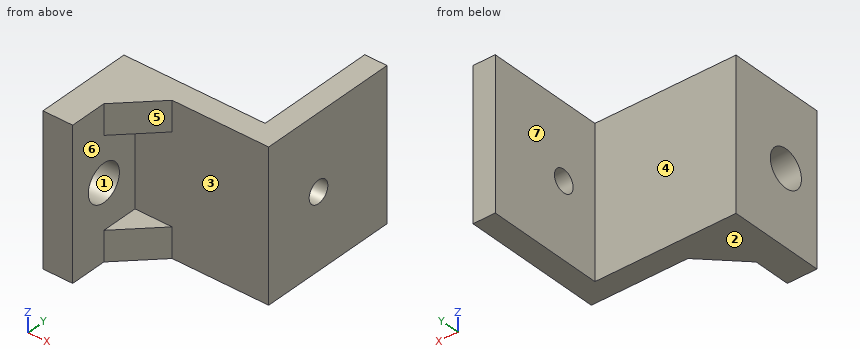
Autodesk Inventor part; units mm, degrees
ref_plane "YZ Plane" through (0, 0, 0) normal (1, 0, 0) x (0, 1, 0)
ref_plane "XZ Plane" through (0, 0, 0) normal (0, 1, 0) x (-1, 0, 0)
ref_plane "XY Plane" through (0, 0, 0) normal (0, 0, 1) x (1, 0, 0)
sketch "Sketch1" plane through (0, 0, 0) normal (0, 0, 1) x (1, 0, 0)
  line L0 (0, 0) -> (22, 0)
  line L1 (22, 0) -> (22, -19)
  line L2 (22, -19) -> (0, -19)
  line L3 (0, -19) -> (0, 0)
  line L4 (3, 0) -> (19, 0)
  line L5 (19, 0) -> (19, -16)
  line L6 (19, -16) -> (3, -16)
  line L7 (3, -16) -> (3, 0)
  dimension "d0" = 22
  dimension "d1" = 19
  dimension "d2" = 3
  dimension "d3" = 3
  dimension "d4" = 3
extrude "Extrusion1" add sketch "Sketch1" along normal blind 20 contours L0 L7 L6 L5 L1 L2 L3
sketch "Sketch4" plane through (3, -16, 0) normal (1, 0, 0) x (0, 0, -1)
  line L0 (-20, 0) -> (-20, 16)
  line L1 (0, 0) -> (-20, 0)
  line L2 (-20, 0) -> (-20, 16)
  line L3 (-20, 16) -> (0, 16)
  line L4 (0, 16) -> (0, 0)
extrude "Extrusion4" cut sketch "Sketch4" against normal through all
sketch "Sketch5" plane through (0, 0, 0) normal (0, 0, -1) x (-1, 0, 0)
  line L0 (0, -19) -> (-22, -19)
  line L1 (0, -19) -> (-4, -19)
  line L2 (-4, -19) -> (-4, -29)
  line L3 (-4, -29) -> (0, -29)
  line L4 (0, -29) -> (0, -19)
  point P0 (0, 0)
  dimension "d17" = 4
  dimension "d18" = 10
extrude "Extrusion5" add sketch "Sketch5" against normal blind 20
sketch "Sketch6" plane through (4, -29, 0) normal (1, 0, 0) x (0, 0, -1)
  line L0 (0, 10) -> (-20, 10)
  line L1 (0, 10) -> (0, 0)
  circle A0 centre (-10, 5) radius 2.5
  point P0 (0, 29)
  dimension "d21" = 5
  dimension "d22" = 10
  dimension "d23" = 5
extrude "Extrusion6" cut sketch "Sketch6" against normal through all
sketch "Sketch7" plane through (0, 0, 0) normal (0, 0, -1) x (-1, 0, 0)
  line L0 (-4, -19) -> (-22, -19)
  line L1 (-4, -29) -> (-4, -19)
  line L2 (-9, -19) -> (-4, -24)
  point P0 (0, 0)
  dimension "d26" = 5
  dimension "d27" = 5
extrude "Extrusion7" add sketch "Sketch7" against normal blind 4
sketch "Sketch8" plane through (0, 0, 20) normal (0, 0, 1) x (1, 0, 0)
  line L0 (4, -19) -> (22, -19)
  line L1 (4, -29) -> (4, -19)
  line L2 (9, -19) -> (4, -24)
  point P0 (0, 0)
  dimension "d30" = 5
  dimension "d31" = 5
extrude "Extrusion8" add sketch "Sketch8" against normal blind 4
sketch "Sketch9" plane through (19, -16, 0) normal (-1, 0, 0) x (0, 0, 1)
  line L0 (0, 16) -> (0, 0)
  line L1 (0, 0) -> (20, 0)
  circle A0 centre (10, 5) radius 1.5
  dimension "d34" = 10
  dimension "d35" = 5
  dimension "d36" = 3
extrude "Extrusion9" cut sketch "Sketch9" against normal through all
equation "\"d3\" = d2"
equation "\"d4\" = d2"
equation "\"d27\" = d26"
equation "\"d30\" = d26"
equation "\"d31\" = d30"
properties part number "LED strip mount v03"
CAD build for the part. Positions are in the model's coordinates, mm. Face numbers are marked on the shaded views. A direction names the side the tool comes from. Round coordinates to 2 decimals unless told otherwise and drop trailing zeros. Loops run counter-clockwise (first coordinate to the right, second up) from the corner with the lowest first, then second, coordinate; pieces in that order, holes last. Notation, with made-up numbers: (-33.75, 23.25) - (-16.75, 23.25) arc R7 cw to (-16.75, 32.25) - close; hole circle Ø6 at (10.5, 8.5). An arc over 180 degrees is marked (long way). Return JSON: item names as keys, results as strings. Group by question number.
Q1. Band-saw the part on B-B on z = 10. Give the cut face in (x, y), plus the area to 3 significant figures.
Q2. Drill centre lines: line 1 along Y through (x, z) = (2.3, 10); line 2 along Y through (x, z) = (21.35, 10); line 3 along X through (y, z) = (-7.25, 4.75). Where is each one in solid material? Low to high. Write a range as [from, to].
Q3. Band-saw the part on C-C on x = 8. Give the cut face in (y, z), plus the area to 3 significant figures.
Q4. Band-saw the part on A-A on y = -11. Give the cut face in (x, z).
Q5. Tool access for the marked faces 5, 6 and 7: list every direction of +Z, -Z, +X, -X, +Y, -Y with a clear straight run to the whole face (end or side of a thin tool).
Q6. Flat gauge pins, fed straight in: pin 1 Ø4 at (x, z) = (8, 7.5) entering from +Y; pin 2 Ø5 at (y, z) = (-10, 7) entering from -X; pin 3 Ø5.5 at (x, z) = (11.5, 11) entering from -Y; pin 4 Ø2 at (x, y) = (17.5, -6) entering from +Z. Where does each tip first touch, or does it go through?
Q7. Band-saw the part on D-D on z = 16.75. Give the cut face in (x, y), plus the area to 4 significant figures.
Q8. Two-plate mould, pull along Z, no slides. Class the marked faces 1, 2, 3 and 4: +Z half, -Z half, draft (parallel to the pull), parting line (faces both ways), or undercut.
Solutions:
{
 "1": {"outline": "(0, -29) - (4, -29) - (4, -26.5) - (0, -26.5) - close; (0, -21.5) - (4, -21.5) - (4, -19) - (22, -19) - (22, -12.5) - (19, -12.5) - (19, -16) - (0, -16) - close; (19, -9.5) - (22, -9.5) - (22, 0) - (19, 0) - close", "area": "125 mm^2"},
 "2": {"line 1": "y = [-29, -26.5], [-21.5, -16]", "line 2": "y = [-19, -12.5], [-9.5, 0]", "line 3": "x = [19, 22]"},
 "3": {"outline": "(-20, 0) - (-16, 0) - (-16, 20) - (-20, 20) - (-20, 16) - (-19, 16) - (-19, 4) - (-20, 4) - close", "area": "68.0 mm^2"},
 "4": {"outline": "(19, 0) - (22, 0) - (22, 8.5) - (19, 8.5) - close; (19, 11.5) - (22, 11.5) - (22, 20) - (19, 20) - close"},
 "5": {"face 5": "+Z, -Z, +X, -Y", "face 6": "+X, -Y", "face 7": "+Z, -Z, -X, +Y"},
 "6": {"pin 1": "stops at y = -16", "pin 2": "stops at x = 19", "pin 3": "stops at y = -19", "pin 4": "passes through"},
 "7": {"outline": "(0, -29) - (4, -29) - (4, -24) - (9, -19) - (22, -19) - (22, 0) - (19, 0) - (19, -16) - (0, -16) - close", "area": "166.5 mm^2"},
 "8": {"face 1": "undercut", "face 2": "-Z half", "face 3": "undercut", "face 4": "draft"}
}
